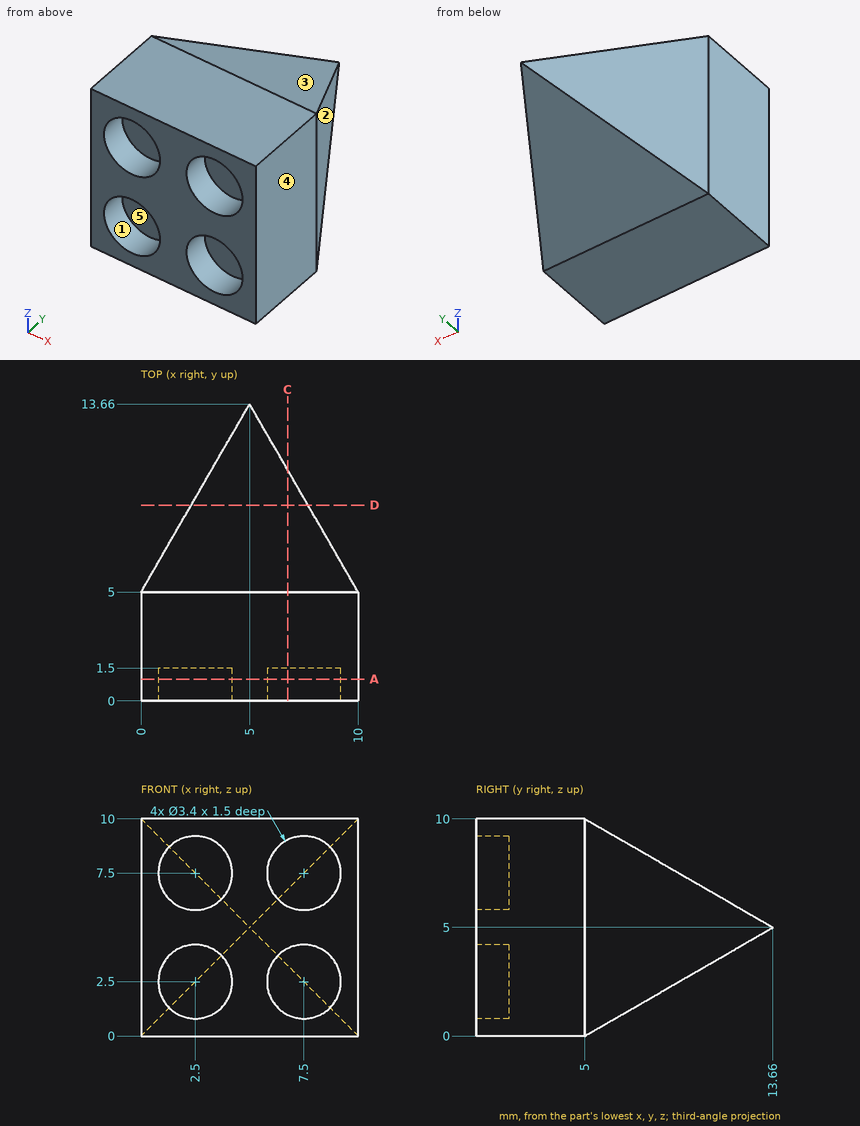
Job drawing, mm, ordinate dimensions from the low corner. One solid piece. A direction names the side the tool comes from. Coordinates: 2 decimals unless noted, no trailing zeros. Order: outer loops, then holes, each group sorted by start corner. A loop starts at its lowest first (then second) coordinate and runs counter-clockwise, first axis right, second up. Notation, with made-up numbers: (56, -26) -> (107, -26) arc R27 ccw to (107, 0) -> close; hole circle Ø9 at (40, 52). An arc over 180 degrees is marked (long way). Put each result on its own line as item: value. Start each with the question number.
(1) Mould opens along X. For the marked faces 3, 4 and 5 say: pulls with the +X half, pulls with the -X half, needs draft (parallel to the pull), parting line crosses it, or undercut.
(2) Band-saw the part on C-C (x = 6.75). Give the cut face in (y, z).
(3) Band-saw the part on D-D (y = 9). Give the cut face in (x, z).
(4) Pin check, flat tips, straight feed: pin 1 Ø3 at (x, z) = (1.5, 4.5) entering from +Y (1 decimal); pin 2 Ø1 at (y, z) = (12, 7) entering from +X; pin 3 Ø1.7 at (x, z) = (2.5, 2.5) entering from -Y; pin 4 Ø2 at (x, z) = (7.5, 7.5) entering from +Y (1 decimal). Stop position of each tip, or through.
(5) Band-saw the part on A-A (y = 1). Give the cut face in (x, z).
(6) Probe line 1 along Z through (x, y) = (7.5, 1); line 2 along Y through (x, z) = (3.75, 2) (1 decimal); line 3 along Z through (x, y) = (7.75, 5.75). List the from-to ranges inside material, lowest first. Write a range as [from, to].
(7) Which spindle directions (+Z, -Z, +X, -X, +Y, -Y) get a long thin tool onto all of the face, cutting with end or side? Do the marked faces 1 and 2. Say none if no direction does.
Determined:
1. face 3: needs draft
1. face 4: pulls with the +X half
1. face 5: undercut
2. outline: (0, 0) -> (5, 0) -> (10.63, 3.25) -> (10.63, 6.75) -> (5, 10) -> (0, 10) -> (0, 9.03) -> (1.5, 9.03) -> (1.5, 5.97) -> (0, 5.97) -> (0, 4.03) -> (1.5, 4.03) -> (1.5, 0.97) -> (0, 0.97) -> close
3. outline: (2.31, 2.31) -> (7.69, 2.31) -> (7.69, 7.69) -> (2.31, 7.69) -> close
4. pin 1: stops at y = 10.2
4. pin 2: passes through
4. pin 3: stops at y = 1.5
4. pin 4: stops at y = 10.6
5. outline: (0, 0) -> (10, 0) -> (10, 10) -> (0, 10) -> close; hole circle Ø3.4 at (2.5, 2.5); hole circle Ø3.4 at (2.5, 7.5); hole circle Ø3.4 at (7.5, 2.5); hole circle Ø3.4 at (7.5, 7.5)
6. line 1: z = [0, 0.8], [4.2, 5.8], [9.2, 10]
6. line 2: y = [1.5, 8.5]
6. line 3: z = [0.43, 9.57]
7. face 1: -Y
7. face 2: +Z, -Z, +X, +Y
